Check sheet for the modelled part. Datum: model origin and axes. Units: mm. A direction names the side the tool comes from. Give positions to 0.01 mm unless a question says otherwise; leave off trailing zeros. Order: outer loops, then holes, each group sorted by start corner. A loop starts at its lowest first (then second) coordinate and runs counter-clockwise, first axis right, second up.
```python
from build123d import *

# Parameters (mm, degrees)
BOSS_EXTRUDE1_DEPTH  = 2.5
M3_CLEARANCE_HOLE1_D = 3.6
SKETCH4_R            = 2.85
SKETCH4_R_2          = 1.1
BOSS_EXTRUDE3_DEPTH  = 45
SKETCH5_W            = 17.6
SKETCH5_H            = 34.321917014
SKETCH5_W_2          = 0.5
CUT_EXTRUDE1_DEPTH   = 23
SKETCH6_R            = 1.65
CUT_EXTRUDE2_DEPTH   = 10
SKETCH7_R            = 1.65
CUT_EXTRUDE3_DEPTH   = 10


with BuildPart() as part:
    # Sketch1 → Boss-Extrude1 (new body)
    with BuildSketch(Plane.XY):
        Polygon((55, -68), (32.25, -12), (26.25, -12), (26.25, 0), (0, 0), (0, -93), (55, -93), align=None)
    boss_extrude1 = extrude(amount=BOSS_EXTRUDE1_DEPTH)

    # Mirror1: Boss-Extrude1 across plane
    add(boss_extrude1.mirror(Plane(origin=(0, 0, 0), x_dir=(0, 0, 1), z_dir=(1, 0, 0))))

    # M3 Clearance Hole1 (through all)
    with Locations(Plane(origin=(0, 0, 0), x_dir=(-1, 0, 0), z_dir=(0, 0, -1))):
        with Locations((0, -10)):
            Hole(M3_CLEARANCE_HOLE1_D / 2)

    # Sketch4 → Boss-Extrude3 (add, symmetric)
    # profile 1 of 2: a face of its own
    with BuildSketch(Plane(origin=(0, 0, 0), x_dir=(0, 0, -1), z_dir=(1, 0, 0))):
        with BuildLine():
            Line((5.200247424, -91.343100719), (0, -85))
            Line((0, -85), (0, -93))
            Line((0, -93), (0.150197759, -93))
            ThreePointArc((0.150197759, -93), (2.107773739, -90.442027677), (5.200247424, -91.343100719))
        make_face()
    # profile 2 of 2: a face of its own
    with BuildSketch(Plane(origin=(0, 0, 0), x_dir=(0, 0, -1), z_dir=(1, 0, 0))):
        with Locations((2.996247653, -93.15)):
            Circle(SKETCH4_R)
        with Locations(Location((2.996247653, -93.15, 0), (0, 0, 180))):
            Circle(SKETCH4_R_2, mode=Mode.SUBTRACT)
    extrude(amount=BOSS_EXTRUDE3_DEPTH, both=True)

    # Sketch5 → Cut-Extrude1 (cut)
    with BuildSketch(Plane(origin=(0, 0, 0), x_dir=(-1, 0, 0), z_dir=(0, 0, -1))):
        with Locations((-18.1, -102.160958507)):
            Rectangle(SKETCH5_W, SKETCH5_H)
        with Locations((18.1, -102.160958507)):
            Rectangle(SKETCH5_W, SKETCH5_H)
        with Locations((-27.15, -102.160958507)):
            Rectangle(SKETCH5_W_2, SKETCH5_H)
        with Locations((-9.05, -102.160958507)):
            Rectangle(SKETCH5_W_2, SKETCH5_H)
        with Locations((9.05, -102.160958507)):
            Rectangle(SKETCH5_W_2, SKETCH5_H)
        with Locations((27.15, -102.160958507)):
            Rectangle(SKETCH5_W_2, SKETCH5_H)
    extrude(amount=CUT_EXTRUDE1_DEPTH, mode=Mode.SUBTRACT)

    # Sketch6 → Cut-Extrude2 (cut)
    with BuildSketch(Plane(origin=(0, 0, 0), x_dir=(-1, 0, 0), z_dir=(0, 0, -1))):
        with Locations((-50, -88)):
            Circle(SKETCH6_R)
        with Locations((-50, -78)):
            Circle(SKETCH6_R)
        with Locations((50, -88)):
            Circle(SKETCH6_R)
        with Locations((50, -78)):
            Circle(SKETCH6_R)
    extrude(amount=-CUT_EXTRUDE2_DEPTH, mode=Mode.SUBTRACT)

    # Sketch7 → Cut-Extrude3 (cut)
    with BuildSketch(Plane(origin=(0, 0, 0), x_dir=(-1, 0, 0), z_dir=(0, 0, -1))):
        with Locations((0, -22)):
            Circle(SKETCH7_R)
        with Locations((0, -32)):
            Circle(SKETCH7_R)
    extrude(amount=-CUT_EXTRUDE3_DEPTH, mode=Mode.SUBTRACT)


solid = part.part
```
(1) Release check for a two-part mould opening along Y. For faces 1 (the face through (43.784, -40.392, 1.232)), 2 (the face through (55, -81, 1)), 3 (the face through (0.12, -94.24, -3.14)) record: released by +Y, released by -Y, zero draft, split by the parting line, or undercut.
Response values:
face 1: released by +Y
face 2: zero draft
face 3: undercut
(2) Cross-section at B-B on y = -10. Enter the section's corners in (x, z), then the cut area to 3 significant figures.
Response values:
outline: (-26.25, 0) - (-1.8, 0) - (-1.8, 2.5) - (-26.25, 2.5) - close; (1.8, 0) - (26.25, 0) - (26.25, 2.5) - (1.8, 2.5) - close
area: 122 mm2
(3) Set-up check for faces 4 (the face through (27.4, -92, -2)), 5 (the face through (0.12, -88.22, -2.64)): record each of +Z, -Z, +X, -X, +Y, -Y from which the full face is reachable in a straight line by a thin tool's end or side.
Response values:
face 4: -Z, +Y, -Y
face 5: -Z, +X, -X, +Y
(4) Cross-section at A-A on x = 0. Enter the section's corners in (y, z).
Response values:
outline: (-93, -0.15) arc R2.85 ccw (long way) to (-91.34, -5.2) - (-85, 0) - (-33.65, 0) - (-33.65, 2.5) - (-93, 2.5) - close; (-30.35, 0) - (-23.65, 0) - (-23.65, 2.5) - (-30.35, 2.5) - close; (-20.35, 0) - (-11.8, 0) - (-11.8, 2.5) - (-20.35, 2.5) - close; (-8.2, 0) - (0, 0) - (0, 2.5) - (-8.2, 2.5) - close; hole circle Ø2.2 at (-93.15, -3)
(5) Material ranges on L1, parallel to X at y = -78, z = 0.55; L2, parallel to X at y = -91, z = -1.75; L3, parallel to Y at x = 0, z = 0.8, recorded low to high.
Response values:
L1: x = -55 to -51.65, -48.35 to 48.35, 51.65 to 55
L2: x = -45 to -27.4, -8.8 to 8.8, 27.4 to 45
L3: y = -93 to -33.65, -30.35 to -23.65, -20.35 to -11.8, -8.2 to 0
(6) Gauge pin test, flat ends, axial feed: pin 1 Ø1.8 at (y, z) = (-90.5, -2) entering from +X; pin 2 Ø1 at (x, z) = (-17, 1) entering from -Y; pin 3 Ø5 at (x, y) = (-12, -66) entering from -Z; pin 4 Ø3 at (x, y) = (0, -10) entering from -Z. Record the tip position at first contact, or that the pin passes through.
Response values:
pin 1: stops at x = 45
pin 2: stops at y = -93
pin 3: stops at z = 0
pin 4: passes through
(7) Cross-section at C-C on y = -78. Enter the section's corners in (x, z).
Response values:
outline: (-55, 0) - (-51.65, 0) - (-51.65, 2.5) - (-55, 2.5) - close; (-48.35, 0) - (48.35, 0) - (48.35, 2.5) - (-48.35, 2.5) - close; (51.65, 0) - (55, 0) - (55, 2.5) - (51.65, 2.5) - close
(8) Cross-section at D-D on x = -50. Enter the section's corners in (y, z).
Response values:
outline: (-93, 0) - (-89.65, 0) - (-89.65, 2.5) - (-93, 2.5) - close; (-86.35, 0) - (-79.65, 0) - (-79.65, 2.5) - (-86.35, 2.5) - close; (-76.35, 0) - (-55.69, 0) - (-55.69, 2.5) - (-76.35, 2.5) - close
